from build123d import *

# Parameters (mm, degrees)
EXTRUDE_1_DEPTH     = 20
SKETCH_2_R          = 2.1
CUT_EXTRUDE_1_DEPTH = 20
SKETCH_3_R          = 4
SKETCH_3_R_2        = 2.1
CUT_EXTRUDE_2_DEPTH = 20


with BuildPart() as part:
    # ｽｹｯﾁ1 → ﾎﾞｽ - 押し出し1 (new body)
    with BuildSketch(Plane.XY):
        Polygon((0, 0), (51.961524227, 0), (51.961524227, 30), align=None)
    extrude(amount=EXTRUDE_1_DEPTH)

    # ｽｹｯﾁ2 → ｶｯﾄ - 押し出し1 (cut)
    with BuildSketch(Plane(origin=(0, 0, 0), x_dir=(-1, 0, 0), z_dir=(0, -1, 0))):
        with Locations(Location((-16.961524227, -10, 0), (0, 0, 180))):
            Circle(SKETCH_2_R)
        with Locations(Location((-41.961524227, -10, 0), (0, 0, 180))):
            Circle(SKETCH_2_R)
    extrude(amount=-CUT_EXTRUDE_1_DEPTH, mode=Mode.SUBTRACT)

    # ｽｹｯﾁ3 → ｶｯﾄ - 押し出し2 (cut)
    # profile 1 of 2: a face of its own
    with BuildSketch(Plane(origin=(0, 5, 0), x_dir=(-1, 0, 0), z_dir=(0, -1, 0))):
        with Locations(Location((-16.961524227, -10, 0), (0, 0, 180))):
            Circle(SKETCH_3_R)
        with Locations(Location((-16.961524227, -10, 0), (0, 0, 180))):
            Circle(SKETCH_3_R_2, mode=Mode.SUBTRACT)
    # profile 2 of 2: a face of its own
    with BuildSketch(Plane(origin=(0, 5, 0), x_dir=(-1, 0, 0), z_dir=(0, -1, 0))):
        with Locations(Location((-41.961524227, -10, 0), (0, 0, 180))):
            Circle(SKETCH_3_R)
        with Locations(Location((-41.961524227, -10, 0), (0, 0, 180))):
            Circle(SKETCH_3_R_2, mode=Mode.SUBTRACT)
    extrude(amount=-CUT_EXTRUDE_2_DEPTH, mode=Mode.SUBTRACT)


solid = part.part
Check sheet for the modelled part. Datum: model origin and axes. Units: mm. A direction names the side the tool comes from. Give positions to 0.01 mm unless a question says otherwise; leave off trailing zeros. Order: outer loops, then holes, each group sorted by start corner. A loop starts at its lowest first (then second) coordinate and runs counter-clockwise, first axis right, second up. Notation, with made-up numbers: (25.5, 78) - (66.5, 78) arc R24 ccw to (66.5, 91) - close; hole circle Ø4 at (76.25, 2). An arc over 180 degrees is marked (long way). Answer as CSV lines item,"result".
1. Go/stop test with flat-tipped pins: P1, Ø5, axis at x = 16.96, z = 10, coming from the +Y side; P2, Ø1.5, axis at x = 35.5, z = 12.5, coming from the +Y side; P3, Ø4, axis at x = 19, z = 9, coming from the +Y side. Record where each tip stops, or that it passes through.
Result sheet:
P1,"y = 5"
P2,"y = 20.93"
P3,"y = 12.12"
2. Section check C-C (z = 17.5). Record the boundary of the cut face in (x, y), then the cut area to 3 significant figures.
Result sheet:
outline,"(0, 0) - (51.96, 0) - (51.96, 30) - close"
area,"779 mm²"
3. Section check B-B (z = 10). Record the boundary of the cut face in (x, y).
Result sheet:
outline,"(0, 0) - (14.86, 0) - (14.86, 5) - (12.96, 5) - (12.96, 7.48) - close; (19.06, 0) - (39.86, 0) - (39.86, 5) - (37.96, 5) - (37.96, 21.92) - (20.96, 12.1) - (20.96, 5) - (19.06, 5) - close; (39.86, 20) - (44.06, 20) - (44.06, 25) - (45.96, 25) - (45.96, 5) - (44.06, 5) - (44.06, 0) - (51.96, 0) - (51.96, 30) - (39.86, 23.01) - close"
4. Section check D-D (x = 39). Record the boundary of the cut face in (y, z).
Result sheet:
outline,"(0, 0) - (22.52, 0) - (22.52, 7.31) - (5, 7.31) - (5, 12.69) - (22.52, 12.69) - (22.52, 20) - (0, 20) - close"
5. Section check A-A (y = 10.5). Record the boundary of the cut face in (x, z).
Result sheet:
outline,"(18.19, 0) - (51.96, 0) - (51.96, 20) - (18.19, 20) - (18.19, 13.81) arc R4 cw to (18.19, 6.19) - close; hole circle Ø8 at (41.96, 10)"
6. Scan lines: probe 1 along Z at (x, y) = (42, 21); probe 2 along Y at (x, z) = (15, 11); probe 3 along Y at (x, z) = (44, 10.75). Record each from-to range of solid material in increasing order. Write a range as from..to.
Result sheet:
probe 1,"0..6, 7.9..12.1, 14..20"
probe 2,"0..5"
probe 3,"0..5, 25..25.4"
7. Tool access check on faces 4 (the face through (42, 20, 10)), 5 (the face through (51.962, 15, 10)), 6 (the face through (37, 9, 20)), 7 (the face through (45.777, 14.86, 11.201)), 8 (the face through (20.777, 7.712, 11.201)). Record the directions out of +Z, -Z, +X, -X, +Y, -Y that give a thin tool (end or side, any length) a straight path to the whole face; none if there is none.
Result sheet:
face 4,"-Y"
face 5,"+Z, -Z, +X, +Y, -Y"
face 6,"+Z, +X, -X, +Y, -Y"
face 7,"none"
face 8,"+Y"
8. Mould release check, pull along Z, two halves, no side actions. Record for faces 1 (the face through (39.864, 2.465, 10.092)), 2 (the face through (37, 9, 0)), 3 (the face through (26, 0, 10)): released by +Z, released by -Z, zero draft, split by the parting line, or undercut.
Result sheet:
face 1,"undercut"
face 2,"released by -Z"
face 3,"zero draft"
